Autodesk Inventor part; units mm, degrees
ref_plane "YZ Plane" through (0, 0, 0) normal (1, 0, 0) x (0, 1, 0)
ref_plane "XZ Plane" through (0, 0, 0) normal (0, 1, 0) x (-1, 0, 0)
ref_plane "XY Plane" through (0, 0, 0) normal (0, 0, 1) x (1, 0, 0)
sketch "Sketch1" plane through (0, 0, 0) normal (0, 1, 0) x (-1, 0, 0)
  line L0 (-55, 62.5) -> (55, 62.5)
  line L1 (55, 62.5) -> (55, -62.5)
  line L2 (55, -62.5) -> (-55, -62.5)
  line L3 (-55, -62.5) -> (-55, 62.5)
  line L4 (-55, 62.5) -> (55, -62.5) construction
  line L5 (55, 62.5) -> (-55, -62.5) construction
  point P0 (0, 0)
  dimension "d0" = 125
  dimension "d1" = 110
extrude "Extrusion1" add sketch "Sketch1" along normal blind 16
sketch "Sketch2" plane through (0, 16, 0) normal (0, 1, 0) x (1, 0, 0)
  line L0 (54, -61.5) -> (-54, -61.5)
  line L1 (-54, -61.5) -> (-54, 61.5)
  line L2 (-54, 61.5) -> (54, 61.5)
  line L3 (54, 61.5) -> (54, -61.5)
  line L4 (54, -61.5) -> (-54, 61.5) construction
  line L5 (-54, -61.5) -> (54, 61.5) construction
  point P0 (0, 0)
  dimension "d4" = 123
  dimension "d5" = 108
extrude "Extrusion2" cut sketch "Sketch2" against normal blind 14
sketch "Sketch3" plane through (0, 2, 0) normal (0, 1, 0) x (1, 0, 0)
  point P0 (0, 0)
sketch "Sketch4" plane through (0, 2, 0) normal (0, 1, 0) x (1, 0, 0)
  line L0 (-17.8843, -36) -> (-42.8843, -36)
  line L1 (-42.8843, -36) -> (-42.8843, 36)
  line L2 (-42.8843, 36) -> (-17.8843, 36)
  line L3 (-17.8843, 36) -> (-17.8843, -36)
  line L4 (-17.8843, -36) -> (-42.8843, 36) construction
  line L5 (-42.8843, -36) -> (-17.8843, 36) construction
  point P0 (0, 0)
  point P1 (-30.3843, 0)
  dimension "d8" = 72
  dimension "d9" = 25
extrude "Extrusion3" cut sketch "Sketch4" against normal blind 14
sketch "Sketch5" plane through (54, 16, -61.5) normal (-1, 0, 0) x (0, 0, 1)
  point P0 (61.5, -16)
sketch "Sketch6" plane through (54, 16, -61.5) normal (-1, 0, 0) x (0, 0, 1)
  line L0 (0, 0) -> (0, -14)
  line L1 (0, -14) -> (123, -14)
  line L2 (0, 0) -> (14, 0)
  line L3 (14, 0) -> (14, -14)
  line L4 (14, -14) -> (0, -14)
  line L5 (0, -14) -> (0, 0)
  point P0 (61.5, -16)
  dimension "d12" = 14
  dimension "d13" = 123
  dimension "d14" = 14
extrude "Extrusion4" cut sketch "Sketch6" against normal blind 14
properties part number "kotak_v2"
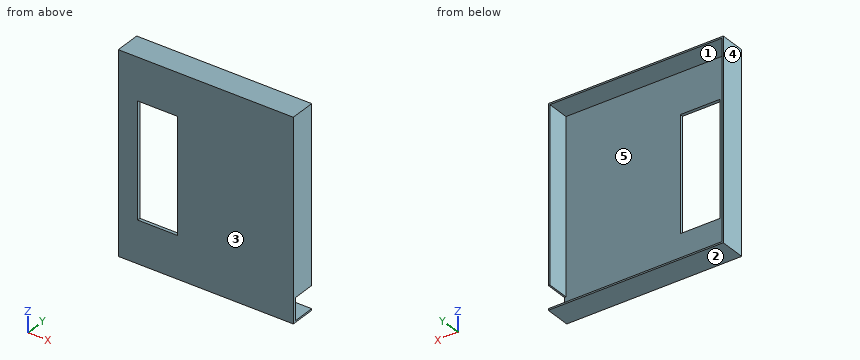
Source: CAD feature listing. Evaluate the final solid. Frame: model axes, mm. Face numbers are marked on the shaded views. A direction names the side the tool comes from. Round coordinates to 2 decimals unless told otherwise and drop trailing zeros. Loops run counter-clockwise (first coordinate to the right, second up) from the corner with the lowest first, then second, coordinate; pieces in that order, holes last.
(1) Section query B-B (x = -28). Output: boundary loops of the cut face in (y, z), and give its area (3 significant figures).
From the geometry:
outline: (0, -62.5) - (16, -62.5) - (16, -61.5) - (2, -61.5) - (2, -36) - (0, -36) - close; (0, 36) - (2, 36) - (2, 61.5) - (16, 61.5) - (16, 62.5) - (0, 62.5) - close
area: 134 mm2
(2) Section query A-A (z = -11.5). Output: boundary loops of the cut face in (x, y).
From the geometry:
outline: (-55, 0) - (-42.88, 0) - (-42.88, 2) - (-54, 2) - (-54, 16) - (-55, 16) - close; (-17.88, 0) - (55, 0) - (55, 16) - (54, 16) - (54, 2) - (-17.88, 2) - close
(3) Contact query for flat-ended pins moving along their axis: pin 1 Ø12 at (x, z) = (-19, 22.5) entering from -Y; pin 2 Ø2 at (x, z) = (20.5, -4) entering from +Y. Output: stop coordinate, or through.
From the geometry:
pin 1: stops at y = 0
pin 2: stops at y = 2
(4) Material intervals for probe 1 along Z at (x, y) = (13, 11.5); probe 2 along X at (y, z) = (10.5, -30); probe 3 along Y at (x, z) = (27, -49), sorted ascending.
From the geometry:
probe 1: z = -62.5 to -61.5, 61.5 to 62.5
probe 2: x = -55 to -54, 54 to 55
probe 3: y = 0 to 2
(5) Pull-direction query (X, two-part tool) for the marked faces 3, 4 and 5; classes: +X half, -X half, draft (parallel to the pull), parting line (faces both ways), or undercut.
From the geometry:
face 3: draft
face 4: -X half
face 5: undercut
(6) Section query D-D (x = 36). Output: boundary loops of the cut face in (y, z).
From the geometry:
outline: (0, -62.5) - (16, -62.5) - (16, -61.5) - (2, -61.5) - (2, 61.5) - (16, 61.5) - (16, 62.5) - (0, 62.5) - close
(7) Section query C-C (y = 13.5). Output: boundary loops of the cut face in (x, z).
From the geometry:
outline: (-55, -62.5) - (55, -62.5) - (55, -61.5) - (-54, -61.5) - (-54, 61.5) - (54, 61.5) - (54, -47.5) - (55, -47.5) - (55, 62.5) - (-55, 62.5) - close
(8) Access query for the marked faces 1 and 2. Directions: +Z, -Z, +X, -X, +Y, -Y. A direction counts if a zero-diameter tool reaches every point of the face in a straight line with its end or side. Return the directions, or none.
From the geometry:
face 1: +Y
face 2: -Z, +X, -X, +Y, -Y
